Part print with two shaded views. Sizes in mm from the minimum x, y, z corner. A direction names the side the tool comes from. Coordinates: 2 decimals unless noted, no trailing zeros. Loops run counter-clockwise (first coordinate to the right, second up) from the corner with the lowest first, then second, coordinate; pieces in that order, holes last. Notation, with made-up numbers: (89.5, 28.25) - (99.5, 28.25) arc R33 ccw to (99.5, 65.25) - close; hole circle Ø6 at (83.5, 53). An arc over 180 degrees is marked (long way). Write each question's results on one line, items separated by ' | '. Start each with the question number.
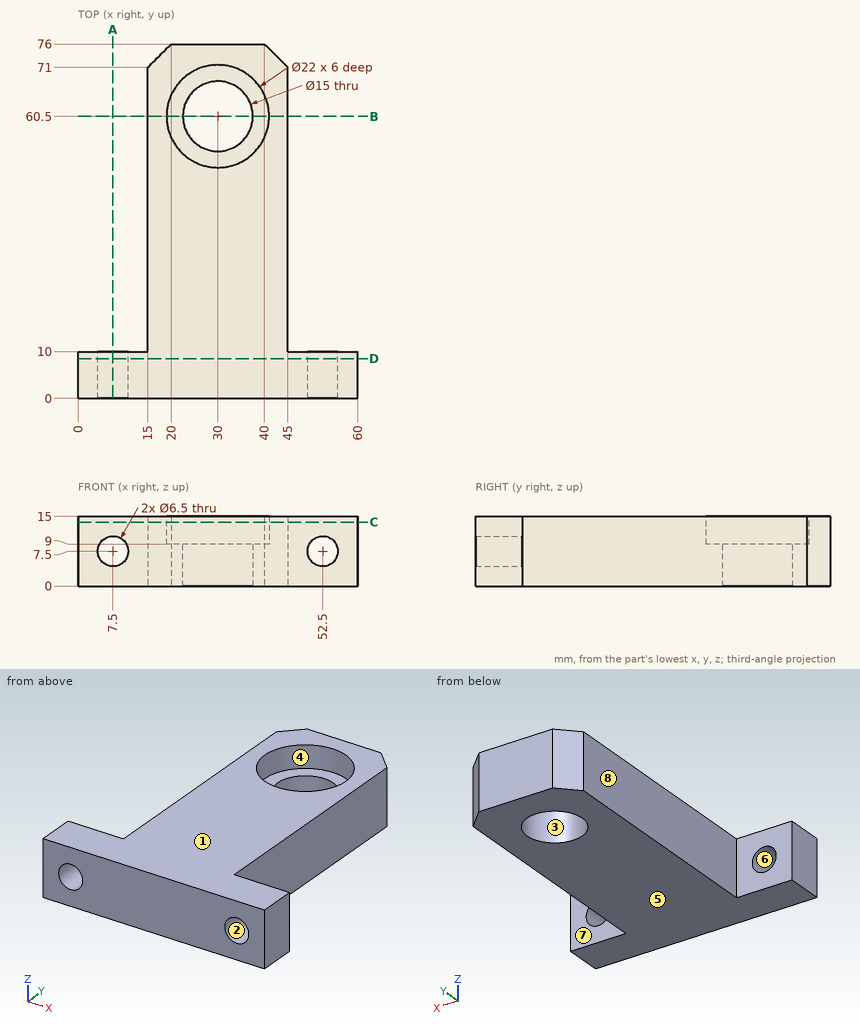
Q1. Mould opens along Z. For the marked faces 1, 2 and 3 say: +Z half, -Z half, draft (parallel to the pull), parting line (faces both ways), or undercut.
Q2. Drill centre lines: L1, parallel to Z at x = 7.5, y = 7.25; L2, parallel to Y at x = 30, z = 13.6; L3, parallel to Y at x = 46, z = 4.25. Where is each one in solid material? Low to high. Write a range as from..to.
Q3. Cut at A-A (x = 7.5). List the corners of the cut face in (y, z).
Q4. Which spindle directions (+Z, -Z, +X, -X, +Y, -Y) get a long thin tool onto all of the face, cutting with end or side? Do the marked faces 4, 5, 6, 7 and 8. Say none if no direction does.
Q5. Cut at C-C (z = 13.75). List the corners of the cut face in (x, y).
Q6. Pin check, flat tips, straight feed: pin 1 (6 mm diameter, centred on y = 36.5, z = 2.5, fed in from -X); pin 2 (7.5 mm diameter, centred on x = 10.5, z = 11, fed in from +Y); pin 3 (4 mm diameter, centred on x = 43.5, z = 12.5, fed in from +Y). Stop position of each tip, or through.
Q7. Cut at B-B (y = 60.5). List the corners of the cut face in (x, z), and give its area (3 significant figures).
Q8. Cut at D-D (y = 8.5). List the corners of the cut face in (x, z), and give its area (3 significant figures).
Check result:
1) face 1: +Z half | face 2: undercut | face 3: draft
2) L1: 0..4.25, 10.75..15 | L2: 0..49.5, 71.5..76 | L3: 0..10
3) outline: (0, 0) - (10, 0) - (10, 4.25) - (0, 4.25) - close; (0, 10.75) - (10, 10.75) - (10, 15) - (0, 15) - close
4) face 4: +Z | face 5: -Z, +X, -X, +Y, -Y | face 6: +Y, -Y | face 7: +Z, -Z, +X, +Y | face 8: +Z, -Z, -X, +Y
5) outline: (0, 0) - (60, 0) - (60, 10) - (45, 10) - (45, 71) - (40, 76) - (20, 76) - (15, 71) - (15, 10) - (0, 10) - close; hole circle Ø22 at (30, 60.5)
6) pin 1: x = 15 | pin 2: y = 10 | pin 3: y = 74.5
7) outline: (15, 0) - (22.5, 0) - (22.5, 9) - (19, 9) - (19, 15) - (15, 15) - close; (37.5, 0) - (45, 0) - (45, 15) - (41, 15) - (41, 9) - (37.5, 9) - close | area: 183 mm²
8) outline: (0, 0) - (60, 0) - (60, 15) - (0, 15) - close; hole circle Ø6.5 at (7.5, 7.5); hole circle Ø6.5 at (52.5, 7.5) | area: 834 mm²
